Work out the finished part from the listing and answer in its coordinate system (mm). A direction names the side the tool comes from. Round coordinates to 2 decimals unless told otherwise and drop trailing zeros. Write each loop counter-clockwise with the first axis right and the second up, starting at its lowest first coordinate (ties: lowest second). Pieces come first, ordered by that corner, then holes.
1. Find section D-D (y = 18). Write down the section's boundary in (x, z), and give its area (4 significant figures).
2. Find section B-B (z = 14.5). Write down the section's boundary in (x, y) (3 decimals).
3. Flat-ended cylindrical pins translate along their axes: pin 1 Ø2 at (x, z) = (46, 28.5) entering from +Y; pin 2 Ø6 at (x, y) = (31, -11) entering from +Z; pin 3 Ø4 at (y, z) = (10, 27) entering from -X; pin 4 Ø11.5 at (x, y) = (53.14, 0) entering from -Z. Find the tip coordinate at first contact, or state that the pin passes through.
4. Straight lines are drawn through the part: probe 1 along Y at (x, z) = (53.5, 29); probe 2 along X at (y, z) = (2.5, 17.5); probe 3 along X at (y, z) = (10, 31.5). For each, find the intervals that lie inside material, in ascending order.
5. Find section A-A (z = 28.5). Write down the section's boundary in (x, y) (3 decimals), and give its area (3 significant figures).
6. Find section C-C (x = -23). Write down the section's boundary in (y, z), and give its area (3 significant figures).
7. Determine the mould class of faces 1 (the face through (-70, 20, 38.1)), 2 (the face through (-9.812, -18.526, 12.522)), 3 (the face through (-55.69, 6.81, 18.78)) for opening direction Y: pulls with the +Y half, pulls with the -Y half, needs draft (parallel to the pull), parting line crosses it, or undercut.
8. A tool of negligible diameter and unlimited length cuts with its end or side. For faces 4 (the face through (56, 6, 31.75)), 5 (the face through (-18, 7, 0)), 6 (the face through (-10, -6.35, 13)), from which of +Z, -Z, +X, -X, +Y, -Y can it reach the whole face along a straight path? Write none if from no direction.
```python
from build123d import *

# Parameters (mm, degrees)
F0_R     = 19.05
F0_R_2   = 6.35
F1_DEPTH = 25.4
F2_DEPTH = 38.1
F3_DEPTH = 31.75


with BuildPart() as f1:
    # F0 (on Top) → F1 (new body)
    with BuildSketch(Plane.XY):
        with BuildLine():
            ThreePointArc((-71.533995, -24.201889), (-55.095046, -16.027055), (-48.459869, 1.091397))
            ThreePointArc((-48.459869, 1.091397), (-54.940362, 18.038734), (-71.075007, 26.338268))
            ThreePointArc((-71.075007, 26.338268), (-99.258822, 1.322061), (-71.533995, -24.201889))
        make_face()
        with Locations((-73.859869, 1.091397)):
            Circle(F0_R, mode=Mode.SUBTRACT)
        with BuildLine():
            ThreePointArc((65.840131, 0), (61.945909, 9.151408), (52.651428, 12.690594))
            ThreePointArc((52.651428, 12.690594), (40.450213, -0.505965), (53.663357, -12.689217))
            ThreePointArc((53.663357, -12.689217), (62.303508, -8.793322), (65.840131, 0))
        make_face()
        with Locations((53.140131, 0)):
            Circle(F0_R_2, mode=Mode.SUBTRACT)
        with BuildLine():
            ThreePointArc((-71.075007, 26.338268), (-54.940362, 18.038734), (-48.459869, 1.091397))
            ThreePointArc((-48.459869, 1.091397), (-55.095046, -16.027055), (-71.533995, -24.201889))
            Line((-71.533995, -24.201889), (53.663357, -12.689217))
            ThreePointArc((53.663357, -12.689217), (40.450213, -0.505965), (52.651428, 12.690594))
            Line((52.651428, 12.690594), (-71.075007, 26.338268))
        make_face()
        with BuildLine():
            ThreePointArc((15.040131, 6.35), (21.390131, 0), (15.040131, -6.35))
            Line((15.040131, -6.35), (-35.759869, -6.35))
            ThreePointArc((-35.759869, -6.35), (-42.109869, 0), (-35.759869, 6.35))
            Line((-35.759869, 6.35), (15.040131, 6.35))
        make_face(mode=Mode.SUBTRACT)
    extrude(amount=F1_DEPTH)

    # F0 (on Top) → F2 (join)
    with BuildSketch(Plane.XY):
        with BuildLine():
            ThreePointArc((-71.533995, -24.201889), (-55.095046, -16.027055), (-48.459869, 1.091397))
            ThreePointArc((-48.459869, 1.091397), (-54.940362, 18.038734), (-71.075007, 26.338268))
            ThreePointArc((-71.075007, 26.338268), (-99.258822, 1.322061), (-71.533995, -24.201889))
        make_face()
        with Locations((-73.859869, 1.091397)):
            Circle(F0_R, mode=Mode.SUBTRACT)
    extrude(amount=F2_DEPTH)

    # F0 (on Top) → F3 (join)
    with BuildSketch(Plane.XY):
        with BuildLine():
            ThreePointArc((65.840131, 0), (61.945909, 9.151408), (52.651428, 12.690594))
            ThreePointArc((52.651428, 12.690594), (40.450213, -0.505965), (53.663357, -12.689217))
            ThreePointArc((53.663357, -12.689217), (62.303508, -8.793322), (65.840131, 0))
        make_face()
        with Locations((53.140131, 0)):
            Circle(F0_R_2, mode=Mode.SUBTRACT)
    extrude(amount=F3_DEPTH)


solid = f1.part
```
Worked answers:
1. outline: (-92.81, 0) - (-82.63, 0) - (-82.63, 38.1) - (-92.81, 38.1) - close; (-65.08, 0) - (4.52, 0) - (4.52, 25.4) - (-54.91, 25.4) - (-54.91, 38.1) - (-65.08, 38.1) - close
1. area: 2,285 mm2
2. outline: (-71.534, -24.202) - (53.663, -12.689) arc R12.7 ccw to (65.84, 0) arc R12.7 ccw to (52.651, 12.691) - (-71.075, 26.338) arc R25.4 ccw (long way) to start; hole circle Ø38.1 at (-73.86, 1.091); hole (-35.76, -6.35) - (15.04, -6.35) arc R6.35 ccw to (15.04, 6.35) - (-35.76, 6.35) arc R6.35 ccw to start; hole circle Ø12.7 at (53.14, 0)
3. pin 1: stops at y = 11.12
3. pin 2: stops at z = 25.4
3. pin 3: stops at x = -98.3
3. pin 4: passes through
4. probe 1: y = -12.69 to -6.34, 6.34 to 12.69
4. probe 2: x = -99.22 to -92.86, -54.86 to -41.6, 20.88 to 47.3, 58.98 to 65.59
4. probe 3: x = -97.65 to -90.7, -57.02 to -50.07, 45.31 to 60.97
5. outline: (-71.534, -24.202) arc R25.4 ccw to (-48.46, 1.091) arc R25.4 ccw to (-71.075, 26.338) arc R25.4 ccw (long way) to start; (53.663, -12.689) arc R12.7 ccw to (65.84, 0) arc R12.7 ccw (long way) to start; hole circle Ø38.1 at (-73.86, 1.091); hole circle Ø12.7 at (53.14, 0)
5. area: 1,270 mm2
6. outline: (-19.74, 0) - (-6.35, 0) - (-6.35, 25.4) - (-19.74, 25.4) - close; (6.35, 0) - (21.04, 0) - (21.04, 25.4) - (6.35, 25.4) - close
6. area: 713 mm2
7. face 1: needs draft
7. face 2: pulls with the -Y half
7. face 3: undercut
8. face 4: +Z, +X, +Y, -Y
8. face 5: -Z, +X, -X, +Y, -Y
8. face 6: +Z, -Z
